Verification items for the finished model (mm, model axes). A direction names the side the tool comes from. Round coordinates to 2 decimals unless told otherwise and drop trailing zeros. Write each loop counter-clockwise with the first axis right and the second up, starting at its lowest first coordinate (ties: lowest second). Pieces come first, ordered by that corner, then holes. Notation, with made-up numbers: M 71,44 L 100,44 A35 cw 100,80 Z; hole C 85.25,85.5 d2. An arc over 180 degrees is marked long. One line per item, written item: value. Start each with the question number.
Item 1: Gauge pin test, flat ends, axial feed: pin 1 (1.2 mm diameter, centred on x = 155, z = 0, fed in from -Y); pin 2 (1.3 mm diameter, centred on x = 171, z = -0.5, fed in from +Y). Record the tip position at first contact, or that the pin passes through.
Item 2: Draft check along X on faces 3 (the face through (205, 0, 0)), 4 (the face through (101, -2.5, 0)), 5 (the face through (137.877, 1.169, -0.093)). Enter one of: +X half, -X half, draft (parallel to the pull), parting line (faces both ways), or undercut.
Item 3: Section check B-B, the plane x = 176.5. Record the cut outline in (y, z).
Item 4: Thickness scan on probe 1 along Z at (x, y) = (170, -1.85); probe 2 along Y at (x, z) = (16, -3); probe 3 along Z at (x, y) = (200, 1.2) (3 decimals). Record the ranges inside material, lowest first. Write a range as from..to.
Item 5: Section check A-A, the plane y = -1.1. State how many separate pieces and enclosed holes the cut face has, then the cut area to 3 significant figures.
Item 6: Tool access check on faces 1 (the face through (62.877, 1.169, -0.093)), 2 (the face through (101, 2.5, 0)). Record the directions out of +Z, -Z, +X, -X, +Y, -Y that give a thin tool (end or side, any length) a straight path to the whole face; none if there is none.
from build123d import *

# Parameters (mm, degrees)
EXTRUDE_1_DEPTH        = 205
SKETCH_3_R             = 1
CUT_EXTRUDE_1_DEPTH    = 25
CUT_EXTRUDE_START      = 2.5
SKETCH_3_3_R           = 2.125
SKETCH_3_3_R_2         = 1
CUT_EXTRUDE_2_DEPTH    = 2.7
PATTERN_LINEAR_1_COUNT = 14
PATTERN_LINEAR_1_PITCH = 15


with BuildPart() as part:
    # 草图2 → 凸台-拉伸1 (new body)
    with BuildSketch(Plane(origin=(0, 0, 0), x_dir=(0, 0, -1), z_dir=(1, 0, 0))):
        Polygon((2.5, 1.15), (3.5, 1.15), (3.5, 2.5), (-3.5, 2.5), (-3.5, 1.15), (-2.5, 1.15), (-2.5, 0.4), (-3.5, 0.4), (-3.5, -2.5), (3.5, -2.5), (3.5, 0.4), (2.5, 0.4), align=None)
    extrude(amount=EXTRUDE_1_DEPTH)

    # 草图3 → 切除-拉伸1 (cut, symmetric)
    with BuildSketch(Plane(origin=(0, 0, 0), x_dir=(1, 0, 0), z_dir=(0, 1, 0))):
        with Locations((5, 0)):
            Circle(SKETCH_3_R)
    cut_extrude_1 = extrude(amount=CUT_EXTRUDE_1_DEPTH, both=True, mode=Mode.SUBTRACT)

    # 草图3<3> → 切除-拉伸2 (cut)
    with BuildSketch(Plane(origin=(0, 0, 0), x_dir=(1, 0, 0), z_dir=(0, 1, 0)).offset(CUT_EXTRUDE_START)):
        with Locations((5, 0)):
            Circle(SKETCH_3_3_R)
        with Locations((5, 0)):
            Circle(SKETCH_3_3_R_2, mode=Mode.SUBTRACT)
    cut_extrude_2 = extrude(amount=-CUT_EXTRUDE_2_DEPTH, mode=Mode.SUBTRACT)

    # 阵列(线性)1: 切除-拉伸1, 切除-拉伸2 ×14
    with Locations(*[(i * PATTERN_LINEAR_1_PITCH, 0, 0) for i in range(1, PATTERN_LINEAR_1_COUNT)]):
        add(cut_extrude_1, mode=Mode.SUBTRACT)
        add(cut_extrude_2, mode=Mode.SUBTRACT)


solid = part.part
Response values:
1. pin 1: passes through
1. pin 2: stops at y = -0.2
2. face 3: +X half
2. face 4: draft
2. face 5: undercut
3. outline: M -2.5,-3.5 L 0.4,-3.5 L 0.4,-2.5 L 1.15,-2.5 L 1.15,-3.5 L 2.5,-3.5 L 2.5,3.5 L 1.15,3.5 L 1.15,2.5 L 0.4,2.5 L 0.4,3.5 L -2.5,3.5 Z
4. probe 1: z = -3.5..-1, 1..3.5
4. probe 2: y = -2.5..0.4, 1.15..2.5
4. probe 3: z = -3.5..-2.125, 2.125..3.5
5. separate pieces: 1
5. enclosed holes: 14
5. area: 1,390 mm2
6. face 1: +Y
6. face 2: +Z, -Z, +X, -X, +Y
